Build history of the part. All positions in model axes, mm. Give positions to 0.01 mm unless a question says otherwise; leave off trailing zeros. Loops run counter-clockwise (first coordinate to the right, second up) from the corner with the lowest first, then second, coordinate; pieces in that order, holes last. Notation, with made-up numbers: (57, 32) -> (79, 32) arc R22 cw to (79, 53) -> close; hole circle Ø5 at (23, 60.5). An arc over 180 degrees is marked (long way). Answer as a JSON object with one key per item and string values. Group by question number.
Q1. Two-plate mould, pull along Z, no slides. Class faces 1 (the cylindrical face through (-70.494, 0.007, -43.264)), 2 (the flat face through (3, -0.5, -52)): pulls with the +Z half, pulls with the -Z half, needs draft (parallel to the pull), parting line crosses it, or undercut.
Q2. Wall check: probe 1 along X at (y, z) = (-0.1, -43); probe 2 along Z at (x, y) = (-64.5, -0.1); probe 3 along X at (y, z) = (-0.1, -39). Give the ranges that are in metal, low to high. Write a range as from..to.
Q3. Band-saw the part on D-D, the plane z = 208. Write the cut outline in (x, y), plus the area to 3 significant figures.
Q4. Band-saw the part on C-C, the plane x = -64.5. Write the cut outline in (y, z), plus the area to 3 significant figures.
Q5. Band-saw the part on A-A, the plane x = 14. Write the cut outline in (y, z).
Q6. Drop flat-ended pins along their axis: pin 1 (11 mm diameter, centred on x = -64.5, z = -43, fed in from +Y); pin 2 (14 mm diameter, centred on x = 64.5, z = -43, fed in from -Y). Give the stop position or say it passes through.
Q7. Band-saw the part on B-B, the plane z = -43. Write the cut outline in (x, y).
Autodesk Inventor part; units mm, degrees
ref_plane "YZ Plane" through (0, 0, 0) normal (1, 0, 0) x (0, 1, 0)
ref_plane "XZ Plane" through (0, 0, 0) normal (0, 1, 0) x (-1, 0, 0)
ref_plane "XY Plane" through (0, 0, 0) normal (0, 0, 1) x (1, 0, 0)
sketch "Esboço1" plane through (0, 0, 0) normal (0, 1, 0) x (-1, 0, 0)
  line L0 (-250, 250) -> (250, 250)
  line L1 (250, 250) -> (250, -250)
  line L2 (250, -250) -> (-250, -250)
  line L3 (-250, -250) -> (-250, 250)
  line L4 (-250, 250) -> (250, -250) construction
  line L5 (250, 250) -> (-250, -250) construction
  point P0 (0, 0)
  dimension "d0" = 500
  dimension "d1" = 500
extrude "Extrusão1" add sketch "Esboço1" along normal mid plane 1
sketch "Esboço2" plane through (0, 0.5, 0) normal (0, 1, 0) x (1, 0, 0)
  line L0 (-105, -12.5) -> (105, -12.5)
  line L1 (105, -12.5) -> (105, 12.5)
  line L2 (105, 12.5) -> (-105, 12.5)
  line L3 (-105, 12.5) -> (-105, -12.5)
  line L4 (-105, -12.5) -> (105, 12.5) construction
  line L5 (105, -12.5) -> (-105, 12.5) construction
  point P0 (0, 0)
  dimension "d4" = 210
  dimension "d5" = 25
extrude "Extrusão2" cut sketch "Esboço2" along normal mid plane 42.75
sketch "Esboço6" plane through (0, 0.5, 0) normal (0, 1, 0) x (1, 0, 0)
  circle A0 centre (-64.5, 43) radius 6
  circle A1 centre (64.5, 43) radius 6
  line L0 (250, 250) -> (-250, 250)
  line L1 (-250, 250) -> (-250, -250)
  line L2 (-64.5, 43) -> (64.5, 43) construction
  line L3 (226, -226) -> (191, -226)
  line L4 (191, -226) -> (191, -201)
  line L5 (201, -191) -> (226, -191)
  line L6 (226, -191) -> (226, -226)
  line L7 (250, -250) -> (250, 250)
  line L8 (-250, -250) -> (250, -250)
  arc A2 (201, -191) -> (191, -201) centre (201, -201) ccw
  point P0 (0, 0)
  point P1 (191, -191)
  dimension "d33" = 12
  dimension "d34" = 12
  dimension "d35" = 207
  dimension "d36" = 185.5
  dimension "d37" = 129
  dimension "d38" = 35
  dimension "d39" = 35
  dimension "d40" = 24
  dimension "d41" = 24
  dimension "d42" = 10
extrude "Extrusão3" cut sketch "Esboço6" against normal up to surface (1 mm away) contours A0 | A1 | L3 L4 A2 L5 L6
properties part number "Chapa - aço galvanizado"
Worked answers:
{
 "1": {"face 1": "undercut", "face 2": "needs draft"},
 "2": {"probe 1": "-250..-70.5, -58.5..58.5, 70.5..250", "probe 2": "-250..-49, -37..-12.5, 12.5..250", "probe 3": "-250..-68.97, -60.03..60.03, 68.97..250"},
 "3": {"outline": "(-250, -0.5) -> (191, -0.5) -> (191, 0.5) -> (-250, 0.5) -> close; (226, -0.5) -> (250, -0.5) -> (250, 0.5) -> (226, 0.5) -> close", "area": "465 mm2"},
 "4": {"outline": "(-0.5, -250) -> (0.5, -250) -> (0.5, -49) -> (-0.5, -49) -> close; (-0.5, -37) -> (0.5, -37) -> (0.5, -12.5) -> (-0.5, -12.5) -> close; (-0.5, 12.5) -> (0.5, 12.5) -> (0.5, 250) -> (-0.5, 250) -> close", "area": "463 mm2"},
 "5": {"outline": "(-0.5, -250) -> (0.5, -250) -> (0.5, -12.5) -> (-0.5, -12.5) -> close; (-0.5, 12.5) -> (0.5, 12.5) -> (0.5, 250) -> (-0.5, 250) -> close"},
 "6": {"pin 1": "through", "pin 2": "y = -0.5"},
 "7": {"outline": "(-250, -0.5) -> (-70.5, -0.5) -> (-70.5, 0.5) -> (-250, 0.5) -> close; (-58.5, -0.5) -> (58.5, -0.5) -> (58.5, 0.5) -> (-58.5, 0.5) -> close; (70.5, -0.5) -> (250, -0.5) -> (250, 0.5) -> (70.5, 0.5) -> close"}
}
